The figure shows three views and two pictorial views of one solid part (mm, origin at its lowest corner). Answer the questions. A direction names the side the tool comes from. Give positions to 0.01 mm unless a question says otherwise; leave off trailing zeros. Write each loop counter-clockwise with the first axis right and the second up, starting at its lowest first coordinate (ties: lowest second). Pieces come first, ordered by that corner, then holes. Notation, with made-up numbers: (89, 17.25) - (111, 17.25) arc R24 cw to (111, 50.25) - close; hole circle Ø2 at (-5, 73). An arc over 180 degrees is marked (long way). One line per question, with ' | ' between items. Start each with the question number.
1. A cutting plane is placed at A-A (x = 10). Determine the outline of the cut face in (y, z).
2. Find the intervals of material crossed by L1, parallel to Z at x = 10, y = 26.5; L2, parallel to Y at x = 10, z = 14; L3, parallel to Z at x = 8.75, y = 15, in increasing order. Write a range as from..to.
3. A cutting plane is placed at B-B (z = 10). Determine the outline of the cut face in (x, y), then the cut area to 3 significant figures.
4. Given P1, Ø1.5, axis at x = 13.5, y = 45.5, coming from the -Z side; P2, Ø5, axis at x = 2.5, y = 38, coming from the -Z side; P3, Ø6, axis at y = 53, z = 13.5, coming from the -X side, each flat-ended and moving along its own axis, determine where each tip first touches the part or whether it passes through.
5. For the marked faces 4 and 5, determine the directions among +Z, -Z, +X, -X, +Y, -Y from which every point of the face is accessible in a straight line to the end or side of a thin tool.
6. The mould has two halves that part along X. Classify the marked faces 1, 2 and 3: +X half, -X half, draft (parallel to the pull), parting line (faces both ways), or undercut.
7. A cutting plane is placed at D-D (y = 62). Determine the outline of the cut face in (x, z).
8. A cutting plane is placed at C-C (y = 13). Determine the outline of the cut face in (x, z), then the cut area to 3 significant figures.
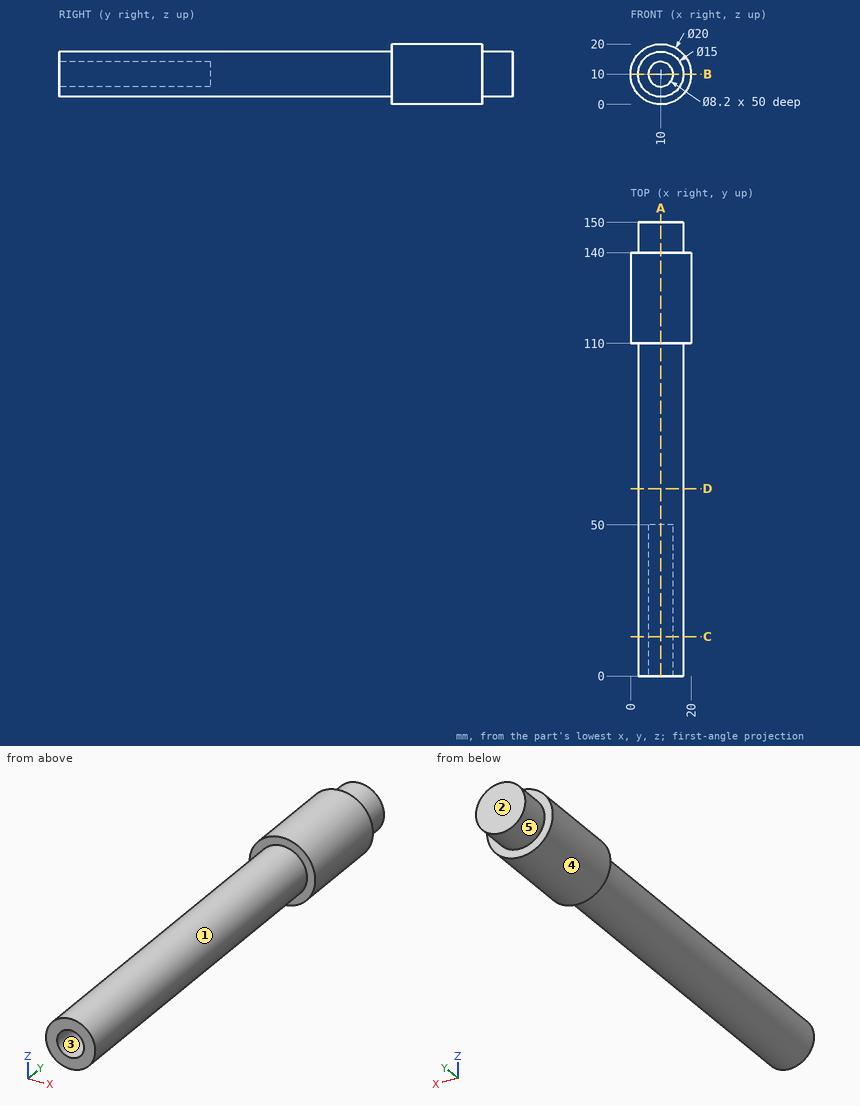
Determined:
1) outline: (0, 2.5) - (110, 2.5) - (110, 0) - (140, 0) - (140, 2.5) - (150, 2.5) - (150, 17.5) - (140, 17.5) - (140, 20) - (110, 20) - (110, 17.5) - (0, 17.5) - (0, 14.1) - (50, 14.1) - (50, 5.9) - (0, 5.9) - close
2) L1: 2.5..5.9, 14.1..17.5 | L2: 50..150 | L3: 2.6..6.1, 13.9..17.4
3) outline: (0, 110) - (2.5, 110) - (2.5, 0) - (5.9, 0) - (5.9, 50) - (14.1, 50) - (14.1, 0) - (17.5, 0) - (17.5, 110) - (20, 110) - (20, 140) - (17.5, 140) - (17.5, 150) - (2.5, 150) - (2.5, 140) - (0, 140) - close | area: 1,990 mm2
4) P1: z = 3.02 | P2: z = 4.41 | P3: x = 2.52
5) face 4: +Y, -Y | face 5: +Y
6) face 1: parting line | face 2: draft | face 3: undercut
7) outline: circle Ø15 at (10, 10)
8) outline: circle Ø15 at (10, 10); hole circle Ø8.2 at (10, 10) | area: 124 mm2
